Check sheet for the modelled part. Datum: model origin and axes. Units: mm. Face numbers are marked on the shaded views. A direction names the side the tool comes from. Coordinates: 2 decimals unless noted, no trailing zeros. Loops run counter-clockwise (first coordinate to the right, second up) from the corner with the lowest first, then second, coordinate; pieces in that order, holes last. Notation, with made-up numbers: (73.25, -5.75) - (102.25, -5.75) arc R34 ccw to (102.25, 33.25) - close; hole circle Ø1 at (54.25, -23). An arc over 180 degrees is marked (long way). Write each question's results on one line, items separated by ' | '. Start each with the question number.
1. Cross-section at D-D (y = -16). Record the cut outline in (x, z).
2. Cross-section at C-C (z = 6.75). Record the cut outline in (x, y), and give its area (3 significant figures).
3. Thickness scan on line 1 (Y direction, x = 0, z = 8); line 2 (Y direction, x = -0.5, z = 6); line 3 (Z direction, x = -2, y = 5). Record the ranges inside material, lowest first. Write a range as [from, to].
4. Tool access check on the marked faces 1 and 2. Record the directions out of +Z, -Z, +X, -X, +Y, -Y that give a thin tool (end or side, any length) a straight path to the whole face; none if there is none.
5. Cross-section at A-A (x = 0). Record the cut outline in (y, z).
6. Gauge pin test, flat ends, axial feed: P1, Ø6, axis at x = -16.5, z = 6.5, coming from the -Y side; P2, Ø8, axis at x = -26.5, y = -0.5, coming from the -Z side; P3, Ø1.5, axis at y = 21.5, z = 8, coming from the +X side; P4, Ø4, axis at y = 24, z = 4, coming from the -X side. Record the tip position at first contact, or that the pin passes through.
7. Draft check along Y on the marked faces 3, 4, 5 and 6. Enter one of: released by +Y, released by -Y, zero draft, split by the parting line, or undercut.
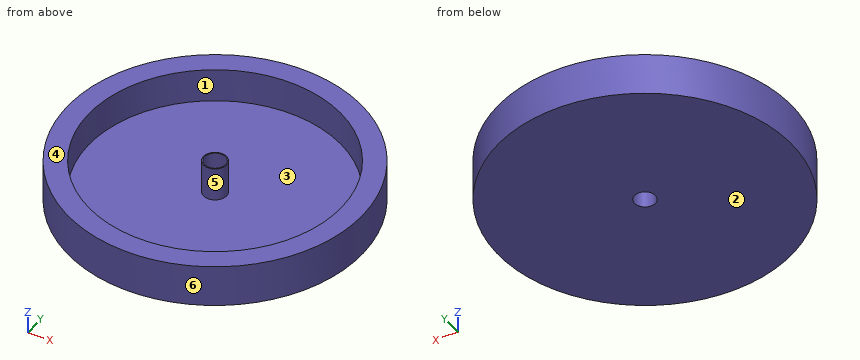
```python
from build123d import *

# Parameters (mm, degrees)
F0_R     = 35
F1_DEPTH = 10
F2_R     = 30
F3_DEPTH = 8
F4_R     = 2.75
F5_DEPTH = 8
F6_R     = 2.5
F7_DEPTH = 10


with BuildPart() as f1:
    # F0 (on Top) → F1 (new body)
    with BuildSketch(Plane.XY):
        Circle(F0_R)
    extrude(amount=F1_DEPTH)

    # F2 (on face) → F3 (cut)
    with BuildSketch(Plane.XY.offset(10)):
        Circle(F2_R)
    extrude(amount=-F3_DEPTH, mode=Mode.SUBTRACT)

    # F4 (on face) → F5 (join)
    with BuildSketch(Plane.XY.offset(2)):
        Circle(F4_R)
    extrude(amount=F5_DEPTH)

    # F6 (on face) → F7 (cut)
    with BuildSketch(Plane.XY.offset(10)):
        Circle(F6_R)
    extrude(amount=-F7_DEPTH, mode=Mode.SUBTRACT)


solid = f1.part
```
Established:
1) outline: (-31.13, 0) - (31.13, 0) - (31.13, 10) - (25.38, 10) - (25.38, 2) - (-25.38, 2) - (-25.38, 10) - (-31.13, 10) - close
2) outline: circle Ø70 at (0, 0); circle Ø5.5 at (0, 0); hole circle Ø60 at (0, 0); hole circle Ø5 at (0, 0) | area: 1,030 mm^2
3) line 1: [-35, -30], [-2.75, -2.5], [2.5, 2.75], [30, 35] | line 2: [-35, -30], [-2.7, -2.45], [2.45, 2.7], [30, 35] | line 3: [0, 2]
4) face 1: +Z | face 2: -Z, +X, -X, +Y, -Y
5) outline: (-35, 0) - (-2.5, 0) - (-2.5, 10) - (-2.75, 10) - (-2.75, 2) - (-30, 2) - (-30, 10) - (-35, 10) - close; (2.5, 0) - (35, 0) - (35, 10) - (30, 10) - (30, 2) - (2.75, 2) - (2.75, 10) - (2.5, 10) - close
6) P1: y = -32.29 | P2: z = 0 | P3: x = 28.19 | P4: x = -27.22
7) face 3: undercut | face 4: zero draft | face 5: undercut | face 6: split by the parting line
